from build123d import *

# Parameters (mm, degrees)
SKETCH_1_W          = 25
SKETCH_1_H          = 37
EXTRUDE_1_DEPTH     = 20
SHELL_1_T           = -2
FILLET_1_R          = 2
CUT_EXTRUDE_1_DEPTH = 43.20485754
CUT_EXTRUDE_2_DEPTH = 43.20485754


with BuildPart() as part:
    # 草图1 → 凸台-拉伸1 (new body)
    with BuildSketch(Plane(origin=(0, 0, 0), x_dir=(1, 0, 0), z_dir=(0, 1, 0))):
        Rectangle(SKETCH_1_W, SKETCH_1_H)
    extrude(amount=EXTRUDE_1_DEPTH)

    # 抽壳1
    shell_1_openings = [part.faces().sort_by_distance(p)[0] for p in [
        (0, 0, 0),
    ]]
    offset(amount=SHELL_1_T, openings=shell_1_openings, kind=Kind.INTERSECTION)

    # 圆角1
    fillet_1_edges = [part.edges().sort_by_distance(p)[0] for p in [
        (12.5, 10, 18.5),
        (-12.5, 10, 18.5),
        (-12.5, 10, -18.5),
        (12.5, 10, -18.5),
    ]]
    fillet(fillet_1_edges, radius=FILLET_1_R)

    # 草图3 → 切除-拉伸1 (cut, through all)
    with BuildSketch(Plane(origin=(0, 0, 16.5), x_dir=(-1, 0, 0), z_dir=(0, 0, -1))):
        Polygon((2.5, 8), (-6.5, 8), (-8.5, 6.5), (-8.5, 4), (-6.5, 2.5), (2.5, 2.5), align=None)
    extrude(amount=-CUT_EXTRUDE_1_DEPTH, mode=Mode.SUBTRACT)

    # 草图3<3> → 切除-拉伸2 (cut, through all)
    with BuildSketch(Plane(origin=(0, 0, 16.5), x_dir=(-1, 0, 0), z_dir=(0, 0, -1))):
        with BuildLine():
            Line((-3.5, 9.8), (3.5, 9.8))
            ThreePointArc((3.5, 9.8), (5.1, 11.4), (3.5, 13))
            Line((3.5, 13), (-3.5, 13))
            ThreePointArc((-3.5, 13), (-5.1, 11.4), (-3.5, 9.8))
        make_face()
    extrude(amount=CUT_EXTRUDE_2_DEPTH, mode=Mode.SUBTRACT)


solid = part.part
For this review, take the finished solid that the model builds, in its own axes (mm). A direction names the side the tool comes from. Give positions to 0.01 mm unless a question says otherwise; leave off trailing zeros. Loops run counter-clockwise (first coordinate to the right, second up) from the corner with the lowest first, then second, coordinate; pieces in that order, holes last. Notation, with made-up numbers: M -13,-9.75 L 2,-9.75 A26 ccw 2,28.25 Z; hole C 33,19.5 d2. An arc over 180 degrees is marked long. Answer as a JSON object with one key per item and string values. Group by question number.
Q1. Add section A-A on x = -0.75. Give the boundary of the cut face in (y, z).
Q2. Add section C-C on x = -9.25. Give the boundary of the cut face in (y, z), and give its area (3 significant figures).
Q3. Insertion check: P1, Ø0.6, axis at y = 4.5, z = 18, coming from the -X side; P2, Ø5, axis at x = 4.5, z = -5, coming from the -Y side; P3, Ø1, axis at x = -1.5, z = -17, coming from the -Y side; P4, Ø1.6, axis at y = 5, z = 17.5, coming from the +X side. Each pin has a flat end and moves straight along its axis. Give the tip position at first contact, or say it passes through.
Q4. For probe 1 along X at (y, z) = (10.5, 3); probe 2 along Z at (x, y) = (-6.5, 9.5); probe 3 along Z at (x, y) = (3, 11.75), list the stretches that pass through material, from the lowest coordinate up. Write a range as [from, to].
Q5. Add section B-B on y = 11.4. Give the boundary of the cut face in (x, z).
Q6. Add section D-D on z = -6.5. Give the boundary of the cut face in (x, y), and give its area (3 significant figures).
Q7. Tool access review of faces 4 (the flat face through (2, 2.5, 17)), 5 (the flat face through (0, 13, -17)), 6 (the flat face through (0, 9, 16.5)): name each direction out of +Z, -Z, +X, -X, +Y, -Y from which nothing blocks a thin tool from reaching the whole face with its end or side.
Q8. Mouldability with a two-part tool opening along Z and no side actions: class faces 1 (the cylindrical face through (11.93, 10.14, -17.9)), 2 (the flat face through (12.5, 10, 0)), 3 (the flat face through (0, 18, 0)) as +Z half, -Z half, draft (parallel to the pull), parting line (faces both ways), or undercut.
Checked values:
{
 "1": {"outline": "M 0,-18.5 L 9.8,-18.5 L 9.8,-16.5 L 0,-16.5 Z; M 0,16.5 L 2.5,16.5 L 2.5,18.5 L 0,18.5 Z; M 8,16.5 L 18,16.5 L 18,-16.5 L 13,-16.5 L 13,-18.5 L 20,-18.5 L 20,18.5 L 8,18.5 Z"},
 "2": {"outline": "M 0,-18.5 L 20,-18.5 L 20,18.5 L 0,18.5 L 0,16.5 L 18,16.5 L 18,-16.5 L 0,-16.5 Z", "area": "146 mm²"},
 "3": {"P1": "x = -12.1", "P2": "y = 18", "P3": "y = 0", "P4": "x = 12.49"},
 "4": {"probe 1": "[-12.5, -10.5], [10.5, 12.5]", "probe 2": "[-18.5, -16.5], [16.5, 18.5]", "probe 3": "[16.5, 18.5]"},
 "5": {"outline": "M -12.5,-16.5 A2 ccw -10.5,-18.5 L -5.1,-18.5 L -5.1,-16.5 L -10.5,-16.5 L -10.5,16.5 L 10.5,16.5 L 10.5,-16.5 L 5.1,-16.5 L 5.1,-18.5 L 10.5,-18.5 A2 ccw 12.5,-16.5 L 12.5,16.5 A2 ccw 10.5,18.5 L -10.5,18.5 A2 ccw -12.5,16.5 Z"},
 "6": {"outline": "M -12.5,0 L -10.5,0 L -10.5,18 L 10.5,18 L 10.5,0 L 12.5,0 L 12.5,20 L -12.5,20 Z", "area": "122 mm²"},
 "7": {"face 4": "+Z", "face 5": "-Z", "face 6": "-Y"},
 "8": {"face 1": "-Z half", "face 2": "draft", "face 3": "undercut"}
}
